from build123d import *

# Parameters (mm, degrees)
PAD_DEPTH          = 2
SKETCH001_W        = 35
SKETCH001_H        = 2
PAD001_DEPTH       = 18
SKETCH002_W        = 44
SKETCH002_H        = 2
PAD002_DEPTH       = 24
CHAMFER_1_SIZE2    = 17.99
CHAMFER_1_SIZE     = 4.49
CHAMFER_2_SIZE2    = 17.99
CHAMFER_2_SIZE     = 4.49
FILLET_R           = 3
SKETCH003_R        = 1.25
POCKET_DEPTH       = 5
SKETCH004_R        = 1.6
POCKET001_DEPTH    = 5
SKETCH005_W        = 1.5
SKETCH005_H        = 14
PAD003_DEPTH       = 35
CHAMFER001_1_SIZE2 = 30
CHAMFER001_1_SIZE  = 10
CHAMFER001_2_SIZE2 = 30
CHAMFER001_2_SIZE  = 10
FILLET001_R        = 3
POCKET002_DEPTH    = 5


with BuildPart() as part:
    # Sketch → Pad (new body)
    with BuildSketch(Plane.XY):
        Polygon((-17.5, -15), (17.5, -15), (17.5, -7), (11, 7), (-11, 7), (-17.5, -7), align=None)
    extrude(amount=PAD_DEPTH)

    # Sketch001 (on Face8 of Pad) → Pad001 (join)
    with BuildSketch(Plane.XY.offset(2)):
        with Locations((0, -14)):
            Rectangle(SKETCH001_W, SKETCH001_H)
    extrude(amount=PAD001_DEPTH)

    # Sketch002 (on Face12 of Pad001) → Pad002 (join)
    with BuildSketch(Plane.XY.offset(20)):
        with Locations((0, -14)):
            Rectangle(SKETCH002_W, SKETCH002_H)
    extrude(amount=PAD002_DEPTH)

    # Chamfer 1
    chamfer_1_edges = [part.edges().sort_by_distance(p)[0] for p in [
        (-17.5, -14, 20),
    ]]
    chamfer_1_side = part.faces().sort_by_distance((-19.75, -14, 20))[0]
    chamfer(chamfer_1_edges, length=CHAMFER_1_SIZE, length2=CHAMFER_1_SIZE2, reference=chamfer_1_side)

    # Chamfer 2
    chamfer_2_edges = [part.edges().sort_by_distance(p)[0] for p in [
        (17.5, -14, 20),
    ]]
    chamfer_2_side = part.faces().sort_by_distance((19.75, -14, 20))[0]
    chamfer(chamfer_2_edges, length=CHAMFER_2_SIZE, length2=CHAMFER_2_SIZE2, reference=chamfer_2_side)

    # Fillet
    fillet_edges = [part.edges().sort_by_distance(p)[0] for p in [
        (22, -14, 44),
        (17.5, -7, 1),
        (11, 7, 1),
        (-11, 7, 1),
        (-17.5, -7, 1),
        (-22, -14, 44),
    ]]
    fillet(fillet_edges, radius=FILLET_R)

    # Sketch003 (on Face1 of Fillet) → Pocket (cut)
    with BuildSketch(Plane(origin=(0, -13, 0), x_dir=(-1, 0, 0), z_dir=(0, 1, 0))):
        with Locations((-19.5, 39)):
            Circle(SKETCH003_R)
        with Locations((19.5, 23)):
            Circle(SKETCH003_R)
    extrude(amount=-POCKET_DEPTH, mode=Mode.SUBTRACT)

    # Sketch004 (on Face16 of Pocket) → Pocket001 (cut)
    with BuildSketch(Plane.XY.offset(2)):
        Circle(SKETCH004_R)
    extrude(amount=-POCKET001_DEPTH, mode=Mode.SUBTRACT)

    # Sketch005 (on Face16 of Pocket001) → Pad003 (join)
    with BuildSketch(Plane.XY.offset(2)):
        with Locations((-8.75, -6)):
            Rectangle(SKETCH005_W, SKETCH005_H)
        with Locations((8.75, -6)):
            Rectangle(SKETCH005_W, SKETCH005_H)
    extrude(amount=PAD003_DEPTH)

    # Chamfer001 1
    chamfer001_1_edges = [part.edges().sort_by_distance(p)[0] for p in [
        (-8.75, 1, 37),
    ]]
    chamfer001_1_side = part.faces().sort_by_distance((-8.75, -6, 37))[0]
    chamfer(chamfer001_1_edges, length=CHAMFER001_1_SIZE, length2=CHAMFER001_1_SIZE2, reference=chamfer001_1_side)

    # Chamfer001 2
    chamfer001_2_edges = [part.edges().sort_by_distance(p)[0] for p in [
        (8.75, 1, 37),
    ]]
    chamfer001_2_side = part.faces().sort_by_distance((8.75, -6, 37))[0]
    chamfer(chamfer001_2_edges, length=CHAMFER001_2_SIZE, length2=CHAMFER001_2_SIZE2, reference=chamfer001_2_side)

    # Fillet001
    fillet001_edges = [part.edges().sort_by_distance(p)[0] for p in [
        (8.75, -9, 37),
        (-8.75, -9, 37),
        (-8.75, 1, 7),
        (8.75, 1, 7),
    ]]
    fillet(fillet001_edges, radius=FILLET001_R)

    # Sketch006 (on Face23 of Fillet001) → Pocket002 (cut)
    with BuildSketch(Plane(origin=(0, -13, 0), x_dir=(-1, 0, 0), z_dir=(0, 1, 0))):
        with BuildLine():
            Line((-6, 2), (-6, 12))
            ThreePointArc((6, 12), (0, 18), (-6, 12))
            Line((6, 2), (6, 12))
            Line((-6, 2), (6, 2))
        make_face()
    extrude(amount=-POCKET002_DEPTH, mode=Mode.SUBTRACT)


solid = part.part
Could you check a few things on this model? Use its own coordinates, in mm. A direction names the side the tool comes from. Give positions to 0.01 mm unless a question says otherwise; leave off trailing zeros. Order: outer loops, then holes, each group sorted by start corner. A loop starts at its lowest first (then second) coordinate and runs counter-clockwise, first axis right, second up.
Item 1: I'm going to push flat-ended pins straight in: pin 1 (2.5 mm diameter, centred on x = 0, y = 0, fed in from -Z); pin 2 (1.6 mm diameter, centred on y = -14, z = 6, fed in from -X); pin 3 (2 mm diameter, centred on y = -14, z = 6.5, fed in from +X); pin 4 (1.5 mm diameter, centred on x = 15.5, z = 25, fed in from +Y). Where does each tip first touch, or does it pass through?
Item 2: If we section it at D-D, the plane x = -7: Write out the boundary of the cut face in (y, z).
Item 3: If we section it at B-B, the plane y = 0: Write out the boundary of the cut face in (x, z).
Item 4: I need wall thicknesses on line 1 (X direction, y = -5, z = 20); line 2 (Y direction, x = -20, z = 27); line 3 (Z direction, x = 13.5, y = -6). Which ranges of each line are inside material? Lowest first, please.
Item 5: If we section it at A-A, the plane z = 39: Write out the boundary of the cut face in (x, y).
Item 6: For faces 1 (the face through (10.719, 6.516, 1.014)), 2 (the face through (-9.5, -8, 15)), 3 (the face through (17.5, -11, 1)), 4 (the face through (-9, -12, 37)), 5 (the face through (-8, -8, 15)), which set-ups out of +Z, -Z, +X, -X, +Y, -Y let a thin tool reach every point of the face, with its end or its side?
Item 7: If we mould it in two halves opening along Z, with no side actions, what happens to faces 6 (the face through (0, -14, 44)), 7 (the face through (14.55, -0.65, 0.99)), 8 (the face through (0, -14, 18))? For each: pulls with the +Z half, pulls with the -Z half, needs draft (parallel to the pull), parting line crosses it, or undercut.
Item 8: If we section it at C-C, the plane x = 0: Write out the boundary of the cut face in (y, z).
Values:
1. pin 1: passes through
1. pin 2: stops at x = -18.7
1. pin 3: stops at x = 18.87
1. pin 4: stops at y = -13
2. outline: (-15, 0) - (7, 0) - (7, 2) - (-13, 2) - (-13, 44) - (-15, 44) - close
3. outline: (-14.25, 0) - (-1.6, 0) - (-1.6, 2) - (-8, 2) - (-8, 10) - (-9.5, 10) - (-9.5, 2) - (-14.25, 2) - close; (1.6, 0) - (14.25, 0) - (14.25, 2) - (9.5, 2) - (9.5, 10) - (8, 10) - (8, 2) - (1.6, 2) - close
4. line 1: x = -9.5 to -8, 8 to 9.5
4. line 2: y = -15 to -13
4. line 3: z = 0 to 2
5. outline: (-22, -15) - (18.25, -15) - (18.25, -13) - (-22, -13) - close; (20.75, -15) - (22, -15) - (22, -13) - (20.75, -13) - close
6. face 1: +Z, -Z, +X, +Y
6. face 2: +Z, -X, +Y
6. face 3: -Z, +X, +Y, -Y
6. face 4: +Z, +X, -X, +Y
6. face 5: +Z, +Y
7. face 6: pulls with the +Z half
7. face 7: needs draft
7. face 8: undercut
8. outline: (-15, 0) - (-1.6, 0) - (-1.6, 2) - (-15, 2) - close; (-15, 18) - (-13, 18) - (-13, 44) - (-15, 44) - close; (1.6, 0) - (7, 0) - (7, 2) - (1.6, 2) - close
